Design review of the part built by this model. Coordinates are the model's own, in mm. Face numbers are marked on the shaded views. Coordinates: 2 decimals unless noted, no trailing zeros. Order: outer loops, then holes, each group sorted by start corner. A loop starts at its lowest first (then second) coordinate and runs counter-clockwise, first axis right, second up. Notation, with made-up numbers: M -12,47.5 L 40,47.5 A30 ccw 40,79.5 Z; hole C 25,-11 d8. An arc over 180 degrees is marked long. Use CSV: the item, a comma, the result in double quotes.
Autodesk Fusion 360 part; units mm, degrees
sketch "NEMA23 bracket front" plane through (0, 0, 0) normal (0, 1, 0) x (1, 0, 0)
  line L0 (-32.5, -3) -> (-32.5, -63)
  line L1 (-32.5, 0) -> (-32.5, -3)
  line L2 (32.5, 0) -> (-32.5, 0)
  line L3 (32.5, -63) -> (32.5, -3)
  line L4 (-32.5, -3) -> (32.5, -3)
  line L5 (-27.5, -68) -> (27.5, -68)
  line L6 (23.55, -15.45) -> (-23.55, -15.45) construction
  line L7 (32.5, -3) -> (32.5, 0)
  circle A0 centre (-23.55, -62.55) radius 2.75
  line L8 (32.5, 0) -> (32.5, -68) construction
  line L9 (23.55, -62.55) -> (-23.55, -62.55) construction
  circle A1 centre (23.55, -15.45) radius 2.75
  line L10 (32.5, -3) -> (-32.5, -3)
  circle A2 centre (0, -39) radius 19.05
  line L11 (-23.55, -62.55) -> (-23.55, -15.45) construction
  line L12 (23.55, -15.45) -> (23.55, -62.55) construction
  circle A3 centre (-23.55, -15.45) radius 2.75
  circle A4 centre (23.55, -62.55) radius 2.75
  line L13 (-32.5, -63) -> (-27.5, -68)
  line L14 (27.5, -68) -> (32.5, -63)
  dimension "d22" = 38.1
  dimension "d23" = 39
  dimension "d24" = 5.5
  dimension "d27" = 47.1
  dimension "d28" = 47.1
  dimension "d29" = 47.1
  dimension "d30" = 5.5
  dimension "d31" = 5.5
  dimension "d32" = 5.5
  dimension "d33" = 68
  dimension "d34" = 32.5
  dimension "d35" = 65
  dimension "d36" = 3
  dimension "d37" = 65
  dimension "d39" = 5.45
  dimension "d46" = 5
  dimension "d47" = 5
extrude "Extrude1" add sketch "NEMA23 bracket front" along normal blind 68 contours L1 L2 L4 L7 L10 makes body 1
extrude "Extrude2" add sketch "NEMA23 bracket front" along normal blind 3 contours L0 L3 L4 L5 L10 L13 L14 bodies 1
sketch "NEMA23 bracket side" plane through (0, 0, 0) normal (1, 0, 0) x (0, 1, 0)
  line L0 (3, 3) -> (24, 3)
  line L1 (24, 3) -> (24, 5)
  line L2 (24, 5) -> (5, 38)
  line L3 (5, 38) -> (3, 38)
  line L4 (3, 38) -> (3, 3)
  dimension "d52" = 21
  dimension "d53" = 35
  dimension "d54" = 2
  dimension "d55" = 2
  dimension "d56" = 3
  dimension "d57" = 3
extrude "Extrude3" add sketch "NEMA23 bracket side" along normal mid plane 65 bodies 1
extrude "Extrude4" cut sketch "NEMA23 bracket side" along normal mid plane 59 bodies 1
sketch "NEMA23 bracket top" plane through (0, 0, 3) normal (0, 0, 1) x (-1, 0, 0)
  line L0 (32.5, -24) -> (29.5, -24)
  line L1 (29.5, -24) -> (29.5, -3)
  line L2 (29.5, -3) -> (-29.5, -3)
  line L3 (-29.5, -3) -> (-29.5, -24)
  line L4 (-29.5, -24) -> (-32.5, -24)
  line L5 (-32.5, -24) -> (-32.5, -68)
  line L6 (-32.5, -68) -> (32.5, -68)
  line L7 (32.5, -68) -> (32.5, -24)
  line L8 (20, -54) -> (-20, -54) construction
  line L9 (-20, -54) -> (-20, -13) construction
  line L10 (-20, -13) -> (20, -13) construction
  line L11 (20, -13) -> (20, -54) construction
  line L12 (32.5, -68) -> (27.5, -68)
  line L13 (32.5, -68) -> (32.5, -63)
  line L14 (27.5, -68) -> (32.5, -63)
  line L15 (-32.5, -68) -> (-27.5, -68)
  line L16 (-32.5, -68) -> (-32.5, -63)
  line L17 (-32.5, -63) -> (-27.5, -68)
  line L18 (22.15, -54) -> (22.15, -13)
  line L19 (17.85, -54) -> (17.85, -13)
  line L20 (-17.85, -54) -> (-17.85, -13)
  line L21 (-22.15, -54) -> (-22.15, -13)
  arc A0 (17.85, -54) -> (22.15, -54) centre (20, -54) ccw
  arc A1 (22.15, -13) -> (17.85, -13) centre (20, -13) ccw
  arc A2 (-17.85, -13) -> (-22.15, -13) centre (-20, -13) ccw
  arc A3 (-22.15, -54) -> (-17.85, -54) centre (-20, -54) ccw
  dimension "d62" = 40
  dimension "d63" = 41
  dimension "d64" = 13
  dimension "d65" = 4.3
  dimension "d66" = 4.3
  dimension "d67" = 4.3
  dimension "d68" = 4.3
  dimension "d69" = 5
  dimension "d70" = 5
  dimension "d71" = 5
  dimension "d72" = 5
extrude "Extrude5" cut sketch "NEMA23 bracket top" against normal blind 5 contours L18 L19 A0 A1 | L20 L21 A2 A3 bodies 1
extrude "Extrude6" cut sketch "NEMA23 bracket top" against normal blind 5 contours L6 L7 L12 L13 L14 | L5 L6 L15 L16 L17 bodies 1
copy_body "Body->Comp1" bodies 1 removing the originals makes body 2 in component "NEMA23 bracket"
component "NEMA23 bracket" placed x (1, 0, 0) y (0, 1, 0) z (0, 0, 1) at (0, 0, 0)
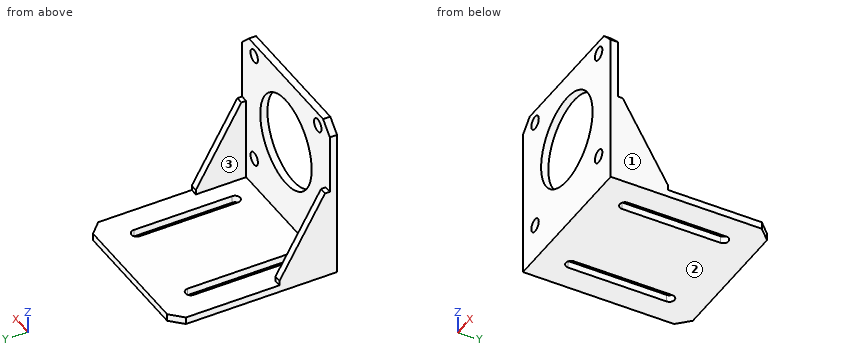
(1) Add section C-C on x = 0. State the section outline as (y, z) points.
The answers:
outline,"M 0,0 L 68,0 L 68,3 L 3,3 L 3,19.95 L 0,19.95 Z; M 0,58.05 L 3,58.05 L 3,68 L 0,68 Z"
(2) Clearance check with flat-ended pins moving along their axes: P1, Ø6, axis at x = 9.5, y = 40.5, coming from the +Z side; P2, Ø5, axis at x = -22.5, z = 9.5, coming from the -Y side; P3, Ø1.6, axis at x = 31.5, y = 4, coming from the +Z side; P4, Ø5, axis at x = -8, z = 18, coming from the +Y side. State where each tip first meets the part, or that it passes through.
The answers:
P1,"stops at z = 3"
P2,"stops at y = 0"
P3,"stops at z = 38"
P4,"stops at y = 3"
(3) Wall thickness on probe 1 along Z at (x, y) = (-23.55, 1.35); probe 2 along X at (y, z) = (1.9, 62.55); probe 3 along X at (y, z) = (1, 62): over which ranges is each line inside the solid? List them lowest first.
The answers:
probe 1,"z = 0 to 12.7, 18.2 to 59.8, 65.3 to 68"
probe 2,"x = -32.5 to -26.3, -20.8 to 20.8, 26.3 to 32.5"
probe 3,"x = -32.5 to -26.24, -20.86 to 20.86, 26.24 to 32.5"
(4) Add section B-B on x = -23.55. State the section outline as (y, z) points.
The answers:
outline,"M 0,0 L 68,0 L 68,3 L 3,3 L 3,12.7 L 0,12.7 Z; M 0,18.2 L 3,18.2 L 3,59.8 L 0,59.8 Z; M 0,65.3 L 3,65.3 L 3,68 L 0,68 Z"
(5) Add section A-A on z = 39. State the section outline as (x, y) points.
The answers:
outline,"M -32.5,0 L -19.05,0 L -19.05,3 L -32.5,3 Z; M 19.05,0 L 32.5,0 L 32.5,3 L 19.05,3 Z"
(6) Add section D-D on z = 53. State the section outline as (x, y) points.
The answers:
outline,"M -32.5,0 L -12.92,0 L -12.92,3 L -32.5,3 Z; M 12.92,0 L 32.5,0 L 32.5,3 L 12.92,3 Z"
(7) The part is to be moulded in two halves that separate along X. For the marked faces 1, 2 and 3, say which applies: pulls with the +X half, pulls with the -X half, needs draft (parallel to the pull), parting line crosses it, or undercut.
The answers:
face 1,"pulls with the +X half"
face 2,"needs draft"
face 3,"undercut"
